Could you check a few things on this model? Use its own coordinates, in mm. A direction names the side the tool comes from. Round coordinates to 2 decimals unless told otherwise and drop trailing zeros. Loops run counter-clockwise (first coordinate to the right, second up) from the corner with the lowest first, then second, coordinate; pieces in that order, holes last. Notation, with made-up numbers: M 40,49.25 L 64,49.25 A31 ccw 64,87.25 Z; hole C 26,75.25 d6. An arc over 180 degrees is marked long. Return JSON: item names as keys, results as strings. Group by question number.
Autodesk Inventor part; units mm, degrees
ref_plane "Work Plane1" through (0, 0, 0) normal (0, 0, 1) x (1, 0, 0)
ref_plane "YZ Plane" through (0, 0, 0) normal (1, 0, 0) x (0, 1, 0)
ref_plane "XZ Plane" through (0, 0, 0) normal (0, 1, 0) x (-1, 0, 0)
ref_plane "Work Plane1" through (0, 0, 0) normal (0, 0, 1) x (1, 0, 0)
sketch "Sketch1" plane through (0, 0, 0) normal (0, 0, 1) x (1, 0, 0)
  line L0 (26.3787, 4.8051) -> (32.3787, 4.8051)
  line L1 (32.3787, 4.8051) -> (32.3787, -2.1949)
  line L2 (32.3787, -2.1949) -> (26.3787, -2.1949)
  line L3 (26.3787, -2.1949) -> (26.3787, 4.8051)
  point P0 (0, 0)
  dimension "d0" = 6
  dimension "d2" = 7
extrude "Extrusion1" add sketch "Sketch1" along normal blind 5
sketch "Sketch2" plane through (32.3787, -2.1949, 0) normal (1, 0, 0) x (0, 0, -1)
  circle A0 centre (-2.5, 3.5) radius 3.1
  line L0 (0, 7) -> (-5, 7)
  line L1 (0, 0) -> (-5, 0)
  line L2 (-2.5, 3.5) -> (-2.5, 7)
  line L3 (-2.5, 3.5) -> (-2.5, 0)
  point P0 (0, 2.1949)
  dimension "d5" = 6.2
extrude "Extrusion2" add sketch "Sketch2" along normal blind 4
sketch "Sketch3" plane through (36.3787, 1.3051, 2.5) normal (1, 0, 0) x (0, 0, -1)
  circle A0 centre (0, 0) radius 3.1
  circle A1 centre (0, 0) radius 1.75
  point P0 (2.5, -1.3051)
  dimension "d9" = 3.5
extrude "Extrusion3" cut sketch "Sketch3" against normal blind 7 contours A1
sketch "Sketch4" plane through (26.3787, -2.1949, 0) normal (-1, 0, 0) x (0, 0, 1)
  line L0 (0, 7) -> (5, 7)
  line L1 (5, 0) -> (2, 0)
  line L2 (2, 0) -> (2, 7)
  line L3 (2, 7) -> (5, 7)
  line L4 (5, 7) -> (5, 0)
  point P0 (0, 2.1949)
  dimension "d13" = 3
extrude "Extrusion4" add sketch "Sketch4" along normal blind 6
properties part number "nanopc_t4_headphone"
1. If we section it at D-D, the plane x = 28.5: Please give me the cut outline in (y, z), then the cut area to 3 significant figures.
2. On a 3-axis mill with a long thin cutter (end or side, diameter ignored), from which of +Z, -Z, +X, -X, +Y, -Y can I reach the whole of each face in a straight line? I mean faces 1 (the face through (26.379, 1, 1)), 2 (the face through (29.379, 1, 3)), 3 (the face through (32.379, -2, 2)), 4 (the face through (26, 1, 5)). Say none if no direction works.
3. I'm going to push flat-ended pins straight in: pin 1 Ø1 at (y, z) = (0, 1) entering from -X; pin 2 Ø1.8 at (x, y) = (22, 1.5) entering from -Z; pin 3 Ø1.8 at (x, y) = (29, 1) entering from -Z. Where does each tip first touch, or does it pass through?
4. If we section it at C-C, the plane y = 1: Please give me the cut outline in (x, z), then the cut area to 3 significant figures.
5. I need wall thicknesses on probe 1 along Y at (x, z) = (32, 2.5); probe 2 along Z at (x, y) = (32, 1.25); probe 3 along Z at (x, y) = (24.5, 0). Which ranges of each line are inside material? Lowest first, please.
6. We'd pull the mould along Z, two halves only. Please class faces 5 (the face through (32.9, 0.6, 0.9)), 6 (the face through (23, 1, 2)), 7 (the face through (32.379, 4.5, 1.9)): +Z half, -Z half, draft (parallel to the pull), parting line (faces both ways), or undercut.
7. If we section it at B-B, the plane x = 32: Please give me the cut outline in (y, z).
8. If we section it at A-A, the plane z = 2.5: Please give me the cut outline in (x, y), then the cut area to 3 significant figures.
Geometry results:
{
 "1": {"outline": "M -2.19,0 L 4.81,0 L 4.81,5 L -2.19,5 Z", "area": "35.0 mm^2"},
 "2": {"face 1": "-Z, -X, +Y, -Y", "face 2": "+X", "face 3": "+X, -Y", "face 4": "+Z, -X, +Y, -Y"},
 "3": {"pin 1": "x = 26.38", "pin 2": "z = 2", "pin 3": "z = 0"},
 "4": {"outline": "M 20.38,2 L 26.38,2 L 26.38,0 L 32.38,0 L 32.38,-0.58 L 36.38,-0.58 L 36.38,0.78 L 29.38,0.78 L 29.38,4.22 L 36.38,4.22 L 36.38,5.58 L 32.38,5.58 L 32.38,5 L 20.38,5 Z", "area": "48.6 mm^2"},
 "5": {"probe 1": "-2.19 to -0.44, 3.06 to 4.81", "probe 2": "0 to 0.75, 4.25 to 5", "probe 3": "2 to 5"},
 "6": {"face 5": "undercut", "face 6": "-Z half", "face 7": "draft"},
 "7": {"outline": "M -2.19,0 L 4.81,0 L 4.81,5 L -2.19,5 Z; hole C 1.31,2.5 d3.5"},
 "8": {"outline": "M 20.38,-2.19 L 32.38,-2.19 L 32.38,-1.79 L 36.38,-1.79 L 36.38,-0.44 L 29.38,-0.44 L 29.38,3.06 L 36.38,3.06 L 36.38,4.41 L 32.38,4.41 L 32.38,4.81 L 20.38,4.81 Z", "area": "84.3 mm^2"}
}
